Geometry check sheet. Reference: the model listing, model coordinates, mm. A direction names the side the tool comes from. Coordinates: 2 decimals unless noted, no trailing zeros. Loops run counter-clockwise (first coordinate to the right, second up) from the corner with the lowest first, then second, coordinate; pieces in that order, holes last. Notation, with made-up numbers: (3.25, 29.5) -> (30.25, 29.5) arc R30 cw to (30.25, 51.5) -> close; hole circle Ø3 at (52.5, -16.75). An arc over 180 degrees is marked (long way). Answer as a JSON object with one key per item and string values.
from build123d import *

# Parameters (mm, degrees)
PAD_DEPTH       = 20
SKETCH001_R     = 5
POCKET_DEPTH    = 4
SKETCH002_R     = 2
POCKET001_DEPTH = 5
FILLET_R        = 1
FILLET001_R     = 1


with BuildPart() as part:
    # Sketch → Pad (new body)
    with BuildSketch(Plane.XY):
        with BuildLine():
            Line((0, 0), (0, 9))
            Line((0, 9), (-12, 9))
            ThreePointArc((-12, 9), (-18.363961, 6.363961), (-21, 0))
            Line((-21, 0), (-14.75, 0))
            ThreePointArc((-9.25, 0), (-12, 2.75), (-14.75, 0))
            Line((-9.25, 0), (0, 0))
        make_face()
    extrude(amount=PAD_DEPTH)

    # Mirrored: part across YZ


with BuildPart() as part_1:
    add(part.part)
    add(part.part.mirror(Plane.YZ))

    # Sketch001 (on Face1 of Mirrored) → Pocket (cut)
    with BuildSketch(Plane(origin=(0, 9, 0), x_dir=(-1, 0, 0), z_dir=(0, 1, 0))):
        with Locations((0, 10)):
            Circle(SKETCH001_R)
    extrude(amount=-POCKET_DEPTH, mode=Mode.SUBTRACT)

    # Sketch002 (on Face13 of Pocket) → Pocket001 (cut)
    with BuildSketch(Plane(origin=(0, 5, 0), x_dir=(-1, 0, 0), z_dir=(0, 1, 0))):
        with Locations((0, 10)):
            Circle(SKETCH002_R)
    extrude(amount=-POCKET001_DEPTH, mode=Mode.SUBTRACT)

    # Fillet
    fillet_edges = [part_1.edges().sort_by_distance(p)[0] for p in [
        (-18.363961, 6.363961, 20),
        (-6, 9, 20),
        (6, 9, 20),
        (18.363961, 6.363961, 20),
        (-18.363961, 6.363961, 0),
        (-6, 9, 0),
        (6, 9, 0),
        (18.363961, 6.363961, 0),
    ]]
    fillet(fillet_edges, radius=FILLET_R)

    # Fillet001
    fillet001_edges = [part_1.edges().sort_by_distance(p)[0] for p in [
        (5, 9, 10),
    ]]
    fillet(fillet001_edges, radius=FILLET001_R)


solid = part_1.part
1. Section check B-B, the plane x = 0. Record the boundary of the cut face in (y, z), then the cut area to 3 significant figures.
Evaluation:
{"outline": "(0, 0) -> (8, 0) arc R1 ccw to (9, 1) -> (9, 4) arc R1 ccw to (8, 5) -> (5, 5) -> (5, 8) -> (0, 8) -> close; (0, 12) -> (5, 12) -> (5, 15) -> (8, 15) arc R1 ccw to (9, 16) -> (9, 19) arc R1 ccw to (8, 20) -> (0, 20) -> close", "area": "119 mm^2"}
2. Mould release check, pull along X, two halves, no side actions. Record for faces 3 (the face through (0, 4, 20)), 4 (the face through (18.294, 6.434, 9.874)), 5 (the face through (0, 3, 12)): released by +X, released by -X, zero draft, split by the parting line, or undercut.
Evaluation:
{"face 3": "zero draft", "face 4": "released by +X", "face 5": "undercut"}
3. Section check D-D, the plane z = 18. Record the boundary of the cut face in (x, y), then the cut area to 3 significant figures.
Evaluation:
{"outline": "(-21, 0) -> (-14.75, 0) arc R2.75 cw to (-9.25, 0) -> (9.25, 0) arc R2.75 cw to (14.75, 0) -> (21, 0) arc R9 ccw to (12, 9) -> (-12, 9) arc R9 ccw to start", "area": "319 mm^2"}
4. Section check C-C, the plane y = 2.25. State how many separate pieces and enclosed holes the cut face has, then the cut area to 3 significant figures.
Evaluation:
{"separate pieces": "3", "enclosed holes": "1", "area": "689 mm^2"}
5. Depth check by flat-ended pin: P1, Ø2, axis at x = -16, z = 15, coming from the +Y side; P2, Ø5, axis at x = 0.5, z = 8, coming from the +Y side; P3, Ø4, axis at y = 7.5, z = 4, coming from the -X side. Enter the tip coordinate at first touch or a pass-through.
Evaluation:
{"P1": "stops at y = 8.49", "P2": "stops at y = 5", "P3": "stops at x = -19.12"}
6. Tool access check on faces 1 (the face through (-11.94, 2.75, 9.86)), 2 (the face through (0.651, 6.521, 14.957)). Record the directions out of +Z, -Z, +X, -X, +Y, -Y that give a thin tool (end or side, any length) a straight path to the whole face; none if there is none.
Evaluation:
{"face 1": "+Z, -Z, -Y", "face 2": "+Y"}
7. Section check A-A, the plane z = 10. Record the boundary of the cut face in (x, y), then the cut area to 3 significant figures.
Evaluation:
{"outline": "(-21, 0) -> (-14.75, 0) arc R2.75 cw to (-9.25, 0) -> (-2, 0) -> (-2, 5) -> (-5, 5) -> (-5, 8) arc R1 ccw to (-6, 9) -> (-12, 9) arc R9 ccw to start; (2, 0) -> (9.25, 0) arc R2.75 cw to (14.75, 0) -> (21, 0) arc R9 ccw to (12, 9) -> (6, 9) arc R1 ccw to (5, 8) -> (5, 5) -> (2, 5) -> close", "area": "259 mm^2"}
8. Thickness scan on probe 1 along X at (y, z) = (2.25, 7.25); probe 2 along X at (y, z) = (0.5, 8.5); probe 3 along Z at (x, y) = (0, 5.85). Record the ranges inside material, lowest first. Write a range as from..to.
Evaluation:
{"probe 1": "x = -20.71..-13.58, -10.42..10.42, 13.58..20.71", "probe 2": "x = -20.99..-14.7, -9.3..-1.32, 1.32..9.3, 14.7..20.99", "probe 3": "z = 0..5, 15..20"}
